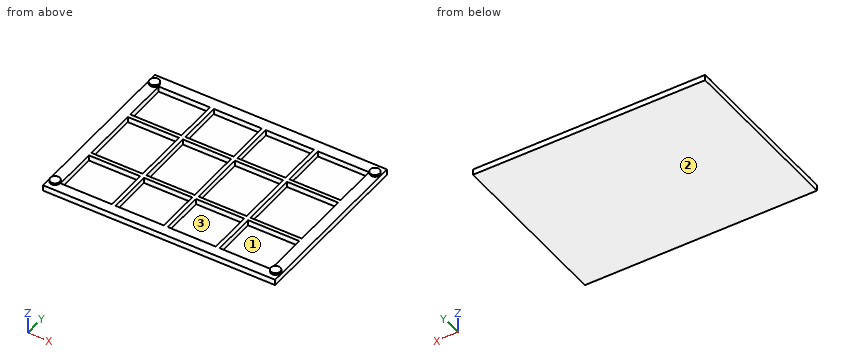
```python
from build123d import *

# Parameters (mm, degrees)
SKETCH2_W           = 1200
SKETCH2_H           = 900
BOSS_EXTRUDE2_DEPTH = 30
SKETCH3_W           = 1087.423470631
SKETCH3_H           = 789.777232946
CUT_EXTRUDE2_DEPTH  = 29
RIB6_REACH          = 1502.3
SKETCH6_WALLS_W     = 20
SKETCH6_WALLS_H     = 3792.377172958
SKETCH6_WALLS_W_2   = 4090.023410643
SKETCH6_WALLS_H_2   = 20
SKETCH7_R           = 25
BOSS_EXTRUDE3_DEPTH = 10


with BuildPart() as part:
    # Sketch2 → Boss-Extrude2 (new body)
    with BuildSketch(Plane.XY):
        with Locations((600, 450)):
            Rectangle(SKETCH2_W, SKETCH2_H)
    extrude(amount=BOSS_EXTRUDE2_DEPTH)

    # Sketch3 → Cut-Extrude2 (cut)
    with BuildSketch(Plane.XY.offset(30)):
        with Locations((600.845585903, 447.040449341)):
            Rectangle(SKETCH3_W, SKETCH3_H)
    extrude(amount=-CUT_EXTRUDE2_DEPTH, mode=Mode.SUBTRACT)

    # Sketch6 walls → Rib6 (add, up to next)
    with BuildSketch(Plane.XY.offset(30), mode=Mode.PRIVATE) as rib6_sk1:
        with Locations((600.845585903, 447.040449341)):
            Rectangle(SKETCH6_WALLS_W, SKETCH6_WALLS_H)
    rib6_tool1 = extrude(rib6_sk1.sketch, amount=-RIB6_REACH, mode=Mode.PRIVATE) - part.part
    # Sketch6 walls → Rib6 (add, up to next)
    with BuildSketch(Plane.XY.offset(30), mode=Mode.PRIVATE) as rib6_sk2:
        with Locations((331.949268904, 447.040449341)):
            Rectangle(SKETCH6_WALLS_W, SKETCH6_WALLS_H)
    rib6_tool2 = extrude(rib6_sk2.sketch, amount=-RIB6_REACH, mode=Mode.PRIVATE) - part.part
    # Sketch6 walls → Rib6 (add, up to next)
    with BuildSketch(Plane.XY.offset(30), mode=Mode.PRIVATE) as rib6_sk3:
        with Locations((600.845585903, 603.473841306)):
            Rectangle(SKETCH6_WALLS_W_2, SKETCH6_WALLS_H_2)
    rib6_tool3 = extrude(rib6_sk3.sketch, amount=-RIB6_REACH, mode=Mode.PRIVATE) - part.part
    # Sketch6 walls → Rib6 (add, up to next)
    with BuildSketch(Plane.XY.offset(30), mode=Mode.PRIVATE) as rib6_sk4:
        with Locations((869.741902901, 447.040449341)):
            Rectangle(SKETCH6_WALLS_W, SKETCH6_WALLS_H)
    rib6_tool4 = extrude(rib6_sk4.sketch, amount=-RIB6_REACH, mode=Mode.PRIVATE) - part.part
    # Sketch6 walls → Rib6 (add, up to next)
    with BuildSketch(Plane.XY.offset(30), mode=Mode.PRIVATE) as rib6_sk5:
        with Locations((600.845585903, 290.607057376)):
            Rectangle(SKETCH6_WALLS_W_2, SKETCH6_WALLS_H_2)
    rib6_tool5 = extrude(rib6_sk5.sketch, amount=-RIB6_REACH, mode=Mode.PRIVATE) - part.part
    add(rib6_tool1.solids().sort_by_distance((600.845585903, 447.040449341, 30))[0])
    add(rib6_tool2.solids().sort_by_distance((331.949268904, 447.040449341, 30))[0])
    add(rib6_tool3.solids().sort_by_distance((600.845585903, 603.473841306, 30))[0])
    add(rib6_tool4.solids().sort_by_distance((869.741902901, 447.040449341, 30))[0])
    add(rib6_tool5.solids().sort_by_distance((600.845585903, 290.607057376, 30))[0])

    # Sketch7 → Boss-Extrude3 (add)
    with BuildSketch(Plane.XY.offset(30)):
        with Locations(Location((30, 850, 0), (0, 0, 180))):
            Circle(SKETCH7_R)
        with Locations(Location((30, 50, 0), (0, 0, 180))):
            Circle(SKETCH7_R)
        with Locations(Location((1170, 50, 0), (0, 0, 180))):
            Circle(SKETCH7_R)
        with Locations(Location((1170, 850, 0), (0, 0, 180))):
            Circle(SKETCH7_R)
    extrude(amount=BOSS_EXTRUDE3_DEPTH)


solid = part.part
```
Verification items for the finished model (mm, model axes). Face numbers are marked on the shaded views. Round coordinates to 2 decimals unless told otherwise and drop trailing zeros. Write each loop counter-clockwise with the first axis right and the second up, starting at its lowest first coordinate (ties: lowest second). Pieces come first, ordered by that corner, then holes.
1. Scan lines: L1, parallel to X at y = 702, z = 5.5; L2, parallel to Y at x = 290, z = 27; L3, parallel to Z at x = 803, y = 115. Record each from-to range of solid material in increasing order.
2. Draft check along Y on the marked faces 1, 2 and 3. Enter one of: +Y half, -Y half, draft (parallel to the pull), parting line (faces both ways), or undercut.
3. Section check D-D on x = 30. Enter the section's corners in (y, z).
4. Section check B-B on y = 202. Enter the section's corners in (x, z), plus the area to 3 significant figures.
5. Section check C-C on z = 22. State how many separate pieces and enclosed holes the cut face has, plus the area to 3 significant figures.
6. Gauge pin test, flat ends, axial feed: P1, Ø1.5, axis at x = 811.5, y = 498.5, coming from the +Z side; P2, Ø10, axis at x = 609.5, y = 703.5, coming from the +Z side. Record the tip position at first contact, or that the pin passes through.
7. Section check A-A on x = 528.5. Enter the section's corners in (y, z).
Answer:
1. L1: x = 0 to 57.13, 321.95 to 341.95, 590.85 to 610.85, 859.74 to 879.74, 1144.56 to 1200
1. L2: y = 0 to 52.15, 280.61 to 300.61, 593.47 to 613.47, 841.93 to 900
1. L3: z = 0 to 1
2. face 1: undercut
2. face 2: draft
2. face 3: undercut
3. outline: (0, 0) - (900, 0) - (900, 30) - (875, 30) - (875, 40) - (825, 40) - (825, 30) - (75, 30) - (75, 40) - (25, 40) - (25, 30) - (0, 30) - close
4. outline: (0, 0) - (1200, 0) - (1200, 30) - (1144.56, 30) - (1144.56, 1) - (879.74, 1) - (879.74, 30) - (859.74, 30) - (859.74, 1) - (610.85, 1) - (610.85, 30) - (590.85, 30) - (590.85, 1) - (341.95, 1) - (341.95, 30) - (321.95, 30) - (321.95, 1) - (57.13, 1) - (57.13, 30) - (0, 30) - close
4. area: 6,200 mm2
5. separate pieces: 1
5. enclosed holes: 12
5. area: 310,000 mm2
6. P1: stops at z = 1
6. P2: stops at z = 30
7. outline: (0, 0) - (900, 0) - (900, 30) - (841.93, 30) - (841.93, 1) - (613.47, 1) - (613.47, 30) - (593.47, 30) - (593.47, 1) - (300.61, 1) - (300.61, 30) - (280.61, 30) - (280.61, 1) - (52.15, 1) - (52.15, 30) - (0, 30) - close
